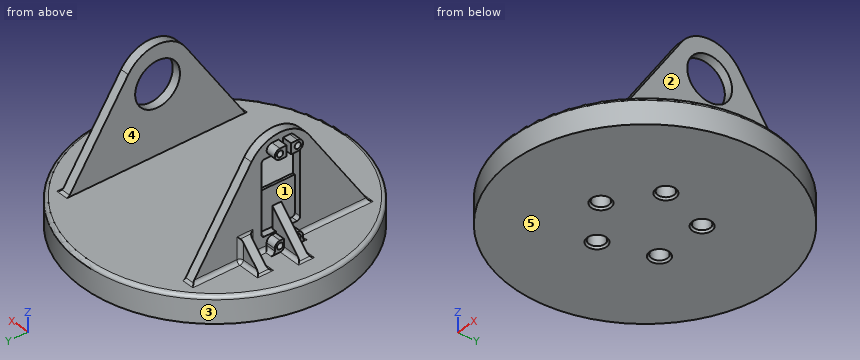
from build123d import *

# Parameters (mm, degrees)
SKETCH1_R           = 75
BASE_PLATE_DEPTH    = 15
SKETCH2_R           = 4.5
DRIVE_HOLES_DEPTH   = 10
CHAMFER1_SIZE       = 1
BASE_START          = 45
BASE_FIN_DEPTH      = 5
BASE_START_2        = 85
BASE_FIN_2_DEPTH    = 5
CUT_EXTRUDE1_REACH  = 122
CUT_EXTRUDE2_REACH  = 122
SKETCH7_R           = 1.75
BOSS_EXTRUDE1_DEPTH = 5.6
SKETCH9_R           = 1.75
CUT_EXTRUDE3_DEPTH  = 5.6
SKETCH10_W          = 4.6
SKETCH10_H          = 2.5
SKETCH10_W_2        = 6
CUT_EXTRUDE4_DEPTH  = 5.6
CUT_EXTRUDE5_DEPTH  = 2.6
BOSS_EXTRUDE2_DEPTH = 1.38
FILLET1_R           = 2
FILLET2_R           = 2
CUT_EXTRUDE6_REACH  = 37
SKETCH13_R          = 12.7
BOSS_EXTRUDE3_DEPTH = 2.5
FILLET3_R           = 2
BOSS_EXTRUDE4_START = 20
BOSS_EXTRUDE4_DEPTH = 2.5
BOSS_EXTRUDE5_START = 20
BOSS_EXTRUDE5_DEPTH = 2.5
FILLET4_R           = 2


with BuildPart() as part:
    # Sketch1 → Base Plate (new body)
    with BuildSketch(Plane.XY):
        Circle(SKETCH1_R)
    extrude(amount=BASE_PLATE_DEPTH)

    # Sketch2 → Drive Holes (cut)
    with BuildSketch(Plane(origin=(0, 0, 0), x_dir=(-1, 0, 0), z_dir=(0, 0, -1))):
        with Locations((0, -25)):
            Circle(SKETCH2_R)
        with Locations((-23.776412907, -7.725424859)):
            Circle(SKETCH2_R)
        with Locations((-14.694631307, 20.225424859)):
            Circle(SKETCH2_R)
        with Locations((14.694631307, 20.225424859)):
            Circle(SKETCH2_R)
        with Locations((23.776412907, -7.725424859)):
            Circle(SKETCH2_R)
    extrude(amount=-DRIVE_HOLES_DEPTH, mode=Mode.SUBTRACT)

    # Chamfer1
    chamfer1_edges = [part.edges().sort_by_distance(p)[0] for p in [
        (28.276412907, -7.725424859, 0),
        (19.194631307, 20.225424859, 0),
        (-10.194631307, 20.225424859, 0),
        (-19.276412907, -7.725424859, 0),
        (4.5, -25, 0),
    ]]
    chamfer(chamfer1_edges, length=CHAMFER1_SIZE)

    # Sketch4 → Base Fin (add)
    with BuildSketch(Plane(origin=(0, 0, 0), x_dir=(0, 0, -1), z_dir=(1, 0, 0)).offset(BASE_START)):
        with BuildLine():
            Line((-15, 50), (-65.791986374, 16.233382914))
            ThreePointArc((-65.791986374, 16.233382914), (-74.493324261, 0), (-65.791986374, -16.233382914))
            Line((-65.791986374, -16.233382914), (-15, -50))
            Line((-15, -50), (-15, 50))
        make_face()
    extrude(amount=-BASE_FIN_DEPTH)

    # Sketch5 → Base Fin 2 (add)
    with BuildSketch(Plane.ZY.offset(-40).offset(BASE_START_2)):
        with BuildLine():
            Line((15, 50), (15, -50))
            Line((15, -50), (65.791986374, -16.233382914))
            ThreePointArc((65.791986374, -16.233382914), (74.493324261, 0), (65.791986374, 16.233382914))
            Line((65.791986374, 16.233382914), (15, 50))
        make_face()
    extrude(amount=-BASE_FIN_2_DEPTH)

    # Sketch6 → Cut-Extrude1 (cut, up to next)
    with BuildSketch(Plane.ZY.offset(45), mode=Mode.PRIVATE) as cut_extrude1_sk1:
        with BuildLine():
            Line((64, 8.832406236), (64, -9.567593764))
            ThreePointArc((64, -9.567593764), (63.487436867, -10.805030631), (62.25, -11.317593764))
            Line((62.25, -11.317593764), (24.05, -11.317593764))
            ThreePointArc((24.05, -11.317593764), (22.812563133, -10.805030631), (22.3, -9.567593764))
            Line((22.3, -9.567593764), (22.3, 8.832406236))
            ThreePointArc((22.3, 8.832406236), (22.812563133, 10.069843103), (24.05, 10.582406236))
            Line((24.05, 10.582406236), (62.25, 10.582406236))
            ThreePointArc((62.25, 10.582406236), (63.487436867, 10.069843103), (64, 8.832406236))
        make_face()
    cut_extrude1_tool1 = extrude(cut_extrude1_sk1.sketch, amount=-CUT_EXTRUDE1_REACH, mode=Mode.PRIVATE) & part.part
    add(cut_extrude1_tool1.solids().sort_by_distance((-45, -0.367594, 43.15))[0], mode=Mode.SUBTRACT)

    # Sketch7 → Cut-Extrude2 (cut, up to next)
    with BuildSketch(Plane.ZY.offset(45), mode=Mode.PRIVATE) as cut_extrude2_sk1:
        with Locations((18.35, 4.632406236)):
            Circle(SKETCH7_R)
    cut_extrude2_tool1 = extrude(cut_extrude2_sk1.sketch, amount=-CUT_EXTRUDE2_REACH, mode=Mode.PRIVATE) & part.part
    add(cut_extrude2_tool1.solids().sort_by_distance((-45, 4.632406, 18.35))[0], mode=Mode.SUBTRACT)
    # Sketch7 → Cut-Extrude2 (cut, up to next)
    with BuildSketch(Plane.ZY.offset(45), mode=Mode.PRIVATE) as cut_extrude2_sk2:
        with Locations((18.35, -5.367593764)):
            Circle(SKETCH7_R)
    cut_extrude2_tool2 = extrude(cut_extrude2_sk2.sketch, amount=-CUT_EXTRUDE2_REACH, mode=Mode.PRIVATE) & part.part
    add(cut_extrude2_tool2.solids().sort_by_distance((-45, -5.367594, 18.35))[0], mode=Mode.SUBTRACT)
    # Sketch7 → Cut-Extrude2 (cut, up to next)
    with BuildSketch(Plane.ZY.offset(45), mode=Mode.PRIVATE) as cut_extrude2_sk3:
        with Locations((67.95, -5.367593764)):
            Circle(SKETCH7_R)
    cut_extrude2_tool3 = extrude(cut_extrude2_sk3.sketch, amount=-CUT_EXTRUDE2_REACH, mode=Mode.PRIVATE) & part.part
    add(cut_extrude2_tool3.solids().sort_by_distance((-45, -5.367594, 67.95))[0], mode=Mode.SUBTRACT)
    # Sketch7 → Cut-Extrude2 (cut, up to next)
    with BuildSketch(Plane.ZY.offset(45), mode=Mode.PRIVATE) as cut_extrude2_sk4:
        with Locations((67.95, 4.632406236)):
            Circle(SKETCH7_R)
    cut_extrude2_tool4 = extrude(cut_extrude2_sk4.sketch, amount=-CUT_EXTRUDE2_REACH, mode=Mode.PRIVATE) & part.part
    add(cut_extrude2_tool4.solids().sort_by_distance((-45, 4.632406, 67.95))[0], mode=Mode.SUBTRACT)

    # Sketch8 → Boss-Extrude1 (add)
    with BuildSketch(Plane.ZY.offset(45)):
        with BuildLine():
            Line((70.95, 4.632406236), (70.95, -5.367593764))
            ThreePointArc((70.95, -5.367593764), (67.95, -8.367593764), (64.95, -5.367593764))
            Line((64.95, -5.367593764), (64.95, 4.632406236))
            ThreePointArc((64.95, 4.632406236), (67.95, 7.632406236), (70.95, 4.632406236))
        make_face()
        with BuildLine():
            Line((15, 7.632406236), (15, 0))
            Line((15, 0), (15, -8.367593764))
            Line((15, -8.367593764), (18.35, -8.367593764))
            ThreePointArc((18.35, -8.367593764), (20.471320344, -7.488914107), (21.35, -5.367593764))
            Line((21.35, -5.367593764), (21.35, 4.632406236))
            ThreePointArc((21.35, 4.632406236), (20.471320344, 6.75372658), (18.35, 7.632406236))
            Line((18.35, 7.632406236), (15, 7.632406236))
        make_face()
    extrude(amount=BOSS_EXTRUDE1_DEPTH)

    # Sketch9 → Cut-Extrude3 (cut)
    with BuildSketch(Plane(origin=(-45, 0, 0), x_dir=(0, 0, -1), z_dir=(1, 0, 0))):
        with Locations((-67.95, -5.367593764)):
            Circle(SKETCH9_R)
        with Locations((-67.95, 4.632406236)):
            Circle(SKETCH9_R)
        with Locations((-18.35, -5.367593764)):
            Circle(SKETCH9_R)
        with Locations((-18.35, 4.632406236)):
            Circle(SKETCH9_R)
    extrude(amount=-CUT_EXTRUDE3_DEPTH, mode=Mode.SUBTRACT)

    # Sketch10 → Cut-Extrude4 (cut)
    with BuildSketch(Plane.ZY.offset(50.6)):
        with Locations((19.05, -0.367593764)):
            Rectangle(SKETCH10_W, SKETCH10_H)
        with Locations((67.95, -0.324654002)):
            Rectangle(SKETCH10_W_2, SKETCH10_H)
    extrude(amount=-CUT_EXTRUDE4_DEPTH, mode=Mode.SUBTRACT)

    # Sketch11 → Cut-Extrude5 (cut)
    with BuildSketch(Plane(origin=(-40, 0, 0), x_dir=(0, 0, -1), z_dir=(1, 0, 0))):
        Polygon((-65.075, -7.027475787), (-65.075, -3.70771174), (-67.95, -2.047829716), (-70.825, -3.70771174), (-70.825, -7.027475787), (-67.95, -8.687357811), align=None)
        Polygon((-65.075, 2.972524213), (-65.075, 6.29228826), (-67.95, 7.952170284), (-70.825, 6.29228826), (-70.825, 2.972524213), (-67.95, 1.312642189), align=None)
        Polygon((-15.475, -7.027475787), (-15.475, -3.70771174), (-18.35, -2.047829716), (-21.225, -3.70771174), (-21.225, -7.027475787), (-18.35, -8.687357811), align=None)
        Polygon((-15.475, 2.972524213), (-15.475, 6.29228826), (-18.35, 7.952170284), (-21.225, 6.29228826), (-21.225, 2.972524213), (-18.35, 1.312642189), align=None)
    extrude(amount=-CUT_EXTRUDE5_DEPTH, mode=Mode.SUBTRACT)

    # Sketch12 → Boss-Extrude2 (add)
    with BuildSketch(Plane(origin=(-40, 0, 0), x_dir=(0, 0, -1), z_dir=(1, 0, 0))):
        with BuildLine():
            Line((-44.572101834, -11.317593764), (-44.572101834, 10.582406236))
            Line((-44.572101834, 10.582406236), (-24.05, 10.582406236))
            ThreePointArc((-24.05, 10.582406236), (-22.812563133, 10.069843103), (-22.3, 8.832406236))
            Line((-22.3, 8.832406236), (-22.3, -9.567593764))
            ThreePointArc((-22.3, -9.567593764), (-22.812563133, -10.805030631), (-24.05, -11.317593764))
            Line((-24.05, -11.317593764), (-44.572101834, -11.317593764))
        make_face()
    extrude(amount=-BOSS_EXTRUDE2_DEPTH)

    # Fillet1
    fillet1_edges = [part.edges().sort_by_distance(p)[0] for p in [
        (-45, -29.183796882, 15),
        (-47.8, -8.367593764, 15),
        (-47.8, 7.632406236, 15),
        (42.5, 50, 15),
        (42.5, -50, 15),
        (45, 0, 15),
        (-42.5, 50, 15),
        (-42.5, -50, 15),
        (-45, 28.816203118, 15),
    ]]
    fillet(fillet1_edges, radius=FILLET1_R)

    # Fillet2
    fillet2_edges = [part.edges().sort_by_distance(p)[0] for p in [
        (-75, 0, 15),
    ]]
    fillet(fillet2_edges, radius=FILLET2_R)

    # Sketch13 → Cut-Extrude6 (cut, up to next)
    with BuildSketch(Plane.ZY.offset(-40), mode=Mode.PRIVATE) as cut_extrude6_sk1:
        with Locations((53.15, -0.367593764)):
            Circle(SKETCH13_R)
    cut_extrude6_tool1 = extrude(cut_extrude6_sk1.sketch, amount=-CUT_EXTRUDE6_REACH, mode=Mode.PRIVATE) & part.part
    add(cut_extrude6_tool1.solids().sort_by_distance((40, -0.367594, 53.15))[0], mode=Mode.SUBTRACT)

    # Sketch15 → Boss-Extrude3 (add, symmetric)
    with BuildSketch(Plane(origin=(0, 0, 0), x_dir=(-1, 0, 0), z_dir=(0, 1, 0))):
        Polygon((42.667233731, 15), (42.667233731, 34.681775652), (62.349009383, 15), align=None)
    extrude(amount=BOSS_EXTRUDE3_DEPTH, both=True)

    # Fillet3
    fillet3_edges = [part.edges().sort_by_distance(p)[0] for p in [
        (-56.474504691, -2.5, 15),
        (-56.474504691, 2.5, 15),
        (-62.349009383, 0, 15),
    ]]
    fillet(fillet3_edges, radius=FILLET3_R)

    # Sketch17 → Boss-Extrude4 (add, symmetric)
    with BuildSketch(Plane(origin=(0, 0, 0), x_dir=(1, 0, 0), z_dir=(0, 1, 0)).offset(BOSS_EXTRUDE4_START)):
        Polygon((-42.667233731, -13), (-42.667233731, -30.724225819), (-60.39145955, -13), align=None)
    extrude(amount=BOSS_EXTRUDE4_DEPTH, both=True)

    # Sketch18 → Boss-Extrude5 (add, symmetric)
    with BuildSketch(Plane(origin=(0, 0, 0), x_dir=(-1, 0, 0), z_dir=(0, 1, 0)).offset(BOSS_EXTRUDE5_START)):
        Polygon((58.39145955, 15), (45, 28.39145955), (45, 15), align=None)
    extrude(amount=BOSS_EXTRUDE5_DEPTH, both=True)

    # Fillet4
    fillet4_edges = [part.edges().sort_by_distance(p)[0] for p in [
        (-45.585786438, 17.5, 15.585786438),
        (-45.585786438, 22.5, 15.585786438),
        (-45, 20, 28.39145955),
        (-58.39145955, 20, 15),
        (-52.695729775, 22.5, 15),
        (-45, 22.5, 22.695729775),
        (-52.695729775, 17.5, 15),
        (-45, 17.5, 22.695729775),
    ]]
    fillet(fillet4_edges, radius=FILLET4_R)


solid = part.part
Work out the finished part from the listing and answer in its coordinate system (mm). Face numbers are marked on the shaded views. A direction names the side the tool comes from. Give positions to 0.01 mm unless a question says otherwise; leave off trailing zeros. Write each loop counter-clockwise with the first axis right and the second up, starting at its lowest first coordinate (ties: lowest second). Pieces come first, ordered by that corner, then holes. Notation, with made-up numbers: (48.5, 55) - (71.5, 55) arc R17 cw to (71.5, 65) - close; hole circle Ø2 at (73, -37.75). An arc over 180 degrees is marked (long way). One line per item, written item: value. Start each with the question number.
1. Find section B-B (z = 37.5). Write down the section's boundary in (x, y).
2. Given pin 1 (6 mm diameter, centred on x = -53.5, y = 31.5, fed in from +Z); pin 2 (5 mm diameter, centred on x = 23.5, y = 1.5, fed in from -Z); pin 3 (7 mm diameter, centred on x = -23.78, y = -7.73, fed in from -Z); pin 4 (1.1 mm diameter, centred on x = -47, y = 2, fed in from +Z), each flat-ended and moving along its own axis, determine where each tip first touches the part or whether it passes through.
3. For the marked faces 1 and 2, determine the directions among +Z, -Z, +X, -X, +Y, -Y from which every point of the face is accessible in a straight line to the end or side of a thin tool.
4. Consider probe 1 along X at (y, z) = (-16, 65.5); probe 2 along Y at (x, z) = (-46, 18); probe 3 along Z at (x, y) = (-4, 48.5). Determine where each line is inside the solid, lowest interval first.
5. For a pull along X with two mould halves and no side action, classify the marked faces 3, 4 and 5 as +X half, -X half, draft (parallel to the pull), parting line (faces both ways), or undercut.
6. Find section A-A (z = 53.15). Write down the section's boundary in (x, y), then the cut area to 3 significant figures.
Geometry results:
1. outline: (-45, -35.04) - (-40, -35.04) - (-40, 35.04) - (-45, 35.04) - (-45, 10.58) - (-41.38, 10.58) - (-41.38, -11.32) - (-45, -11.32) - close; (40, -35.04) - (45, -35.04) - (45, 35.04) - (40, 35.04) - close
2. pin 1: z = 15
2. pin 2: z = 0
2. pin 3: z = 10
2. pin 4: z = 70.95
3. face 1: none
3. face 2: +Z, +X, +Y, -Y
4. probe 1: -45 to -40, 40 to 45
4. probe 2: -8.37 to -7.08, -3.65 to 2.92, 6.35 to 7.63, 17.23 to 22.77
4. probe 3: 0 to 15
5. face 3: parting line
5. face 4: undercut
5. face 5: draft
6. outline: (-45, -24.64) - (-40, -24.64) - (-40, -11.32) - (-45, -11.32) - close; (-45, 10.58) - (-40, 10.58) - (-40, 24.64) - (-45, 24.64) - close; (40, -24.64) - (45, -24.64) - (45, -13.07) - (40, -13.07) - close; (40, 12.33) - (45, 12.33) - (45, 24.64) - (40, 24.64) - close
6. area: 256 mm2
